```python
from build123d import *

# Parameters (mm, degrees)
SKETCH1_W           = 20
SKETCH1_H           = 20
BOSS_EXTRUDE1_DEPTH = 20
CUT_EXTRUDE1_DEPTH  = 2
CUT_EXTRUDE2_DEPTH  = 2
CUT_EXTRUDE3_DEPTH  = 2


with BuildPart() as part:
    # Sketch1 → Boss-Extrude1 (new body)
    with BuildSketch(Plane(origin=(0, 0, 0), x_dir=(1, 0, 0), z_dir=(0, 1, 0))):
        Rectangle(SKETCH1_W, SKETCH1_H)
    extrude(amount=BOSS_EXTRUDE1_DEPTH)

    # Sketch2 → Cut-Extrude1 (cut)
    with BuildSketch(Plane.XY.offset(10)):
        Polygon((-5.076923077, 15.961538462), (-5.076923077, 17.5), (6.269230769, 17.5), (-2.700120192, 4.038461538), (6.076923077, 4.038461538), (6.076923077, 2.5), (-6.038461538, 2.5), (2.930889423, 15.961538462), align=None)
    extrude(amount=-CUT_EXTRUDE1_DEPTH, mode=Mode.SUBTRACT)

    # Sketch3 → Cut-Extrude2 (cut)
    with BuildSketch(Plane(origin=(10, 0, 0), x_dir=(0, 0, -1), z_dir=(1, 0, 0))):
        Polygon((-6.442307692, 17.5), (-4.405048077, 17.5), (0.288461538, 11.439302885), (4.984975962, 17.5), (7.019230769, 17.5), (1.307091346, 10.123197115), (7.211538462, 2.5), (5.177283654, 2.5), (0.288461538, 8.810096154), (-4.597355769, 2.5), (-6.634615385, 2.5), (-0.727163462, 10.123197115), align=None)
    extrude(amount=-CUT_EXTRUDE2_DEPTH, mode=Mode.SUBTRACT)

    # Sketch4 → Cut-Extrude3 (cut)
    with BuildSketch(Plane(origin=(0, 20, 0), x_dir=(1, 0, 0), z_dir=(0, 1, 0))):
        Polygon((-5.480769231, 7.5), (-3.939302885, 7.5), (0.003004808, 1.0546875), (3.939302885, 7.5), (5.480769231, 7.5), (0.673076923, -0.369591346), (0.673076923, -7.5), (-0.673076923, -7.5), (-0.673076923, -0.369591346), align=None)
    extrude(amount=-CUT_EXTRUDE3_DEPTH, mode=Mode.SUBTRACT)


solid = part.part
```
Source: CAD feature listing. Evaluate the final solid. Frame: model axes, mm. A direction names the side the tool comes from. Give positions to 0.01 mm unless a question says otherwise; leave off trailing zeros. Loops run counter-clockwise (first coordinate to the right, second up) from the corner with the lowest first, then second, coordinate; pieces in that order, holes last. Notation, with made-up numbers: (-20, 68.5) -> (28, 68.5) arc R12 cw to (28, 88.5) -> close; hole circle Ø4 at (70.5, -19.75). An arc over 180 degrees is marked (long way). Use a Markdown table: item, result. Add a question column.
(1) Pull-direction query (X, two-part tool) for faces 1 (the face through (0.4, 18, -1.1)), 2 (the face through (10, 10, 2)), 3 (the face through (9.01, 13.86, -4.2)); classes: +X half, -X half, draft (parallel to the pull), parting line (faces both ways), or undercut.
(2) Section query A-A (x = -2). Output: boundary loops of the cut face in (y, z), then the cut area to 3 significant figures.
(3) Section query B-B (z = 1.5). Output: boundary loops of the cut face in (x, y).
(4) Section query D-D (z = -6). Output: boundary loops of the cut face in (x, y).
(5) Access query for faces 4 (the face through (0, 0, 0)), 5 (the face through (9.01, 14.51, 2.09)), 6 (the face through (-2, 20, 0)), 7 (the face through (-5, 19, -7.5)), 8 (the face through (6.077, 3, 9)). Directions: +Z, -Z, +X, -X, +Y, -Y. A direction counts if a zero-diameter tool reaches every point of the face in a straight line with its end or side. Return the directions, or none.
(6) Ray query, line 1 (X direction, y = 18.75, z = -2); line 2 (Y direction, x = -4.75, z = 8.5); line 3 (Z direction, x = -2.75, y = 19). Return the intervals inside material, ascending.
(7) Section query C-C (y = 15.25). Output: boundary loops of the cut face in (x, z).
Checked values:
| question | item | result |
|---|---|---|
| 1 | face 1 | undercut |
| 1 | face 2 | +X half |
| 1 | face 3 | draft |
| 2 | outline | (0, -10) -> (20, -10) -> (20, -4.33) -> (18, -4.33) -> (18, -1.8) -> (20, -1.8) -> (20, 10) -> (17.5, 10) -> (17.5, 8) -> (15.96, 8) -> (15.96, 10) -> (8.56, 10) -> (8.56, 8) -> (5.09, 8) -> (5.09, 10) -> (4.04, 10) -> (4.04, 8) -> (2.5, 8) -> (2.5, 10) -> (0, 10) -> close |
| 2 | area | 382 mm^2 |
| 3 | outline | (-10, 0) -> (10, 0) -> (10, 6.5) -> (8, 6.5) -> (8, 9.13) -> (10, 9.13) -> (10, 11.12) -> (8, 11.12) -> (8, 13.75) -> (10, 13.75) -> (10, 20) -> (0.67, 20) -> (0.67, 18) -> (-0.67, 18) -> (-0.67, 20) -> (-10, 20) -> close |
| 4 | outline | (-10, 0) -> (10, 0) -> (10, 2.5) -> (8, 2.5) -> (8, 4.06) -> (10, 4.06) -> (10, 16.18) -> (8, 16.18) -> (8, 17.5) -> (10, 17.5) -> (10, 20) -> (4.56, 20) -> (4.56, 18) -> (3.02, 18) -> (3.02, 20) -> (-3.02, 20) -> (-3.02, 18) -> (-4.56, 18) -> (-4.56, 20) -> (-10, 20) -> close |
| 5 | face 4 | +Z, -Z, +X, -X, -Y |
| 5 | face 5 | +X |
| 5 | face 6 | +Z, -Z, +X, -X, +Y |
| 5 | face 7 | +Y |
| 5 | face 8 | +Z |
| 6 | line 1 | -10 to -2.12, -0.58 to 0.58, 2.12 to 10 |
| 6 | line 2 | 0 to 2.5, 4.43 to 15.96, 17.5 to 20 |
| 6 | line 3 | -10 to -5.56, -3.03 to 10 |
| 7 | outline | (-10, -10) -> (10, -10) -> (10, -5.28) -> (8, -5.28) -> (8, -3.24) -> (10, -3.24) -> (10, 2.66) -> (8, 2.66) -> (8, 4.7) -> (10, 4.7) -> (10, 10) -> (4.77, 10) -> (4.77, 8) -> (2.46, 8) -> (2.46, 10) -> (-10, 10) -> close |
